from build123d import *

# Parameters (mm, degrees)
SKETCH_1_W          = 24.73
SKETCH_1_H          = 45.23
EXTRUDE_1_DEPTH     = 32
CHAMFER_1_SIZE      = 2
EXTRUDE_2_DEPTH     = 1
SKETCH_3_R          = 1
CUT_EXTRUDE_1_DEPTH = 4
SKETCH_4_R          = 9.975
EXTRUDE_3_DEPTH     = 2.2
SKETCH_5_R          = 2
SKETCH_5_R_2        = 1
CUT_EXTRUDE_2_DEPTH = 3
SKETCH_6_W          = 20.33
SKETCH_6_H          = 12
EXTRUDE_4_DEPTH     = 2
CHAMFER_2_SIZE      = 2
SKETCH_7_W          = 22.33
SKETCH_7_H          = 5
CUT_EXTRUDE_3_DEPTH = 2
SKETCH_8_R          = 3
EXTRUDE_5_DEPTH     = 4.1
CUT_EXTRUDE_START   = -4
SKETCH_9_R          = 1
CUT_EXTRUDE_4_DEPTH = 4
FILLET_1_R          = 1


with BuildPart() as part:
    # 스케치1 → 보스-돌출1 (new body)
    with BuildSketch(Plane.XY):
        Rectangle(SKETCH_1_W, SKETCH_1_H)
    extrude(amount=EXTRUDE_1_DEPTH)

    # 모따기1
    chamfer_1_edges = [part.edges().sort_by_distance(p)[0] for p in [
        (-12.365, 22.615, 16),
        (12.365, 22.615, 16),
    ]]
    chamfer(chamfer_1_edges, length=CHAMFER_1_SIZE)

    # 스케치2 → 보스-돌출2 (add)
    with BuildSketch(Plane.XY.offset(32)):
        with BuildLine():
            Line((-7, -22.615), (7, -22.615))
            Line((7, -22.615), (7, 2.753205655))
            ThreePointArc((7, 2.753205655), (0, 0.5), (-7, 2.753205655))
            Line((-7, 2.753205655), (-7, -22.615))
        make_face()
    extrude(amount=EXTRUDE_2_DEPTH)

    # 스케치3 → 컷-돌출1 (cut)
    with BuildSketch(Plane.XY.offset(32)):
        with Locations((-10.25, 3.885)):
            Circle(SKETCH_3_R)
        with Locations((-10.25, -16.615)):
            Circle(SKETCH_3_R)
        with Locations((10.25, -16.615)):
            Circle(SKETCH_3_R)
        with Locations((10.25, 3.885)):
            Circle(SKETCH_3_R)
    extrude(amount=-CUT_EXTRUDE_1_DEPTH, mode=Mode.SUBTRACT)

    # 스케치4 → 보스-돌출3 (add)
    with BuildSketch(Plane.XY.offset(32)):
        with Locations((0, 12.5)):
            Circle(SKETCH_4_R)
    extrude(amount=EXTRUDE_3_DEPTH)

    # 스케치5 → 컷-돌출2 (cut)
    with BuildSketch(Plane.XY.offset(34.2)):
        with Locations((0, 12.5)):
            Circle(SKETCH_5_R)
        with Locations((0, 19.5)):
            Circle(SKETCH_5_R_2)
        with Locations((7, 12.5)):
            Circle(SKETCH_5_R_2)
        with Locations((0, 5.5)):
            Circle(SKETCH_5_R_2)
        with Locations((-7, 12.5)):
            Circle(SKETCH_5_R_2)
    extrude(amount=-CUT_EXTRUDE_2_DEPTH, mode=Mode.SUBTRACT)

    # 스케치6 → 보스-돌출4 (add)
    with BuildSketch(Plane(origin=(0, 0, 0), x_dir=(-1, 0, 0), z_dir=(0, 0, -1))):
        with Locations((0, -12.115)):
            Rectangle(SKETCH_6_W, SKETCH_6_H)
    extrude(amount=EXTRUDE_4_DEPTH)

    # 모따기2
    chamfer_2_edges = [part.edges().sort_by_distance(p)[0] for p in [
        (0, -6.115, -2),
    ]]
    chamfer(chamfer_2_edges, length=CHAMFER_2_SIZE - 0.0001)  # a hair under: the kernel refuses the full size

    # 스케치7 → 컷-돌출3 (cut)
    with BuildSketch(Plane(origin=(0, 0, 0), x_dir=(-1, 0, 0), z_dir=(0, 0, -1))):
        with Locations((0, -3.615)):
            Rectangle(SKETCH_7_W, SKETCH_7_H)
    extrude(amount=-CUT_EXTRUDE_3_DEPTH, mode=Mode.SUBTRACT)

    # 스케치8 → 보스-돌출5 (add)
    with BuildSketch(Plane(origin=(0, 0, 0), x_dir=(-1, 0, 0), z_dir=(0, 0, -1))):
        with Locations(Location((0, 12.5, 0), (0, 0, 180))):
            Circle(SKETCH_8_R)
    extrude(amount=EXTRUDE_5_DEPTH)

    # 스케치9 → 컷-돌출4 (cut)
    with BuildSketch(Plane(origin=(0, 0, 0), x_dir=(-1, 0, 0), z_dir=(0, 0, -1)).offset(CUT_EXTRUDE_START)):
        with Locations(Location((-10.25, 3.885, 0), (0, 0, 180))):
            Circle(SKETCH_9_R)
        with Locations(Location((10.25, 3.885, 0), (0, 0, 180))):
            Circle(SKETCH_9_R)
        with Locations((-10.25, -20.615)):
            Circle(SKETCH_9_R)
        with Locations((10.25, -20.615)):
            Circle(SKETCH_9_R)
    extrude(amount=CUT_EXTRUDE_4_DEPTH, mode=Mode.SUBTRACT)

    # 필렛1
    fillet_1_edges = [part.edges().sort_by_distance(p)[0] for p in [
        (12.365, -22.615, 16),
        (-12.365, -22.615, 16),
    ]]
    fillet(fillet_1_edges, radius=FILLET_1_R)


solid = part.part
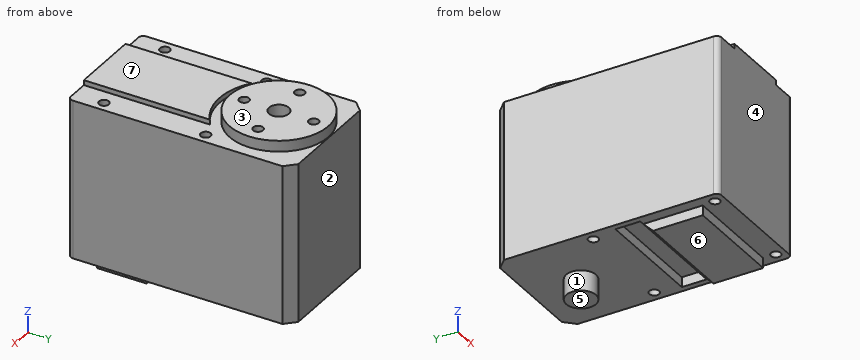
CAD build for the part. Positions are in the model's coordinates, mm. Face numbers are marked on the shaded views. A direction names the side the tool comes from. Give positions to 0.01 mm unless a question says otherwise; leave off trailing zeros. Loops run counter-clockwise (first coordinate to the right, second up) from the corner with the lowest first, then second, coordinate; pieces in that order, holes last. Notation, with made-up numbers: M -30,56.5 L -24,56.5 A27 ccw -24,91.5 Z; hole C 67.25,37 d8. An arc over 180 degrees is marked long. One line per question, with ' | ' between items. Start each with the question number.
1. 3-axis set-ups, long thin cutter, end or side, ignore diameter. For the marked faces 5, 6 and 7: which of +Z, -Z, +X, -X, +Y, -Y reach the whole face in a straight line?
2. Saw through at C-C on z = -1. Give the cut face in (x, y) (3 decimals), plus the area to 3 significant figures.
3. Saw through at B-B on y = -3. Give the cut face in (x, z) (3 decimals), plus the area to 3 significant figures.
4. Probe L1, parallel to Y at x = 10.25, z = 1.2 (3 decimals); L2, parallel to Y at x = -10.25, z = 2.6 (3 decimals); L3, parallel to Z at x = -3, y = -19. List the from-to ranges inside material, lowest first. Write a range as from..to.
5. Two-plate mould, pull along Y, no slides. Class the marked faces 1, 2, 3 and 4: pulls with the +Y half, pulls with the -Y half, needs draft (parallel to the pull), parting line crosses it, or undercut.
6. Flat gauge pins, fed straight in: pin 1 (2.5 mm diameter, centred on x = 10.25, y = -20.615, fed in from +Z); pin 2 (1.2 mm diameter, centred on x = 0, y = 5.5, fed in from +Z); pin 3 (1.6 mm diameter, centred on x = 10.5, y = -20.5, fed in from -Z). Where does each tip first touch, or does it go through?
7. Saw through at D-D on y = 12.5. Give the cut face in (x, z) (3 decimals).
Result sheet:
1) face 5: -Z, +X, -X, +Y, -Y | face 6: -Z, +X, -X, -Y | face 7: +Z, +X, -X, -Y
2) outline: M -10.165,-18.115 L 10.165,-18.115 L 10.165,-7.115 L -10.165,-7.115 Z; C 0,12.5 d6 | area: 252 mm^2
3) outline: M -12.365,0 L -11.165,0 L -11.165,2 L 11.165,2 L 11.165,0 L 12.365,0 L 12.365,32 L 7,32 L 7,33 L -7,33 L -7,32 L -12.365,32 Z | area: 761 mm^2
4) L1: y = -22.615..-21.615, -19.615..-6.115, -1.115..2.885, 4.885..22.615 | L2: y = -22.615..-21.615, -19.615..2.885, 4.885..22.615 | L3: z = 0..33
5) face 1: undercut | face 2: pulls with the +Y half | face 3: needs draft | face 4: pulls with the -Y half
6) pin 1: stops at z = 32 | pin 2: stops at z = 31.2 | pin 3: stops at z = 0
7) outline: M -12.365,0 L -3,0 L -3,-4.1 L 3,-4.1 L 3,0 L 12.365,0 L 12.365,32 L 9.975,32 L 9.975,34.2 L 8,34.2 L 8,31.2 L 6,31.2 L 6,34.2 L 2,34.2 L 2,31.2 L -2,31.2 L -2,34.2 L -6,34.2 L -6,31.2 L -8,31.2 L -8,34.2 L -9.975,34.2 L -9.975,32 L -12.365,32 Z
